```python
from build123d import *

# Parameters (mm, degrees)
SKETCH1_R           = 1.5
SKETCH1_R_2         = 1.7
SKETCH1_R_3         = 2
SKETCH1_W           = 32
SKETCH1_H           = 15
BOSS_EXTRUDE1_DEPTH = 10


with BuildPart() as part:
    # Sketch1 → Boss-Extrude1 (new body)
    with BuildSketch(Plane.XY):
        Polygon((-86.049704166, 116.333921241), (48.950295834, 116.333921241), (48.950295834, 81.333921241), (56.950295834, 81.333921241), (56.950295834, 79.313921241), (130.950295834, 79.313921241), (130.950295834, 81.333921241), (138.950295834, 81.333921241), (138.950295834, 116.333921241), (273.950295834, 116.333921241), (273.950295834, -113.666078759), (138.950295834, -113.666078759), (138.950295834, -78.666078759), (130.950295834, -78.666078759), (130.950295834, -76.646078759), (56.950295834, -76.646078759), (56.950295834, -78.666078759), (48.950295834, -78.666078759), (48.950295834, -113.666078759), (-86.049704166, -113.666078759), (-86.049704166, -78.666078759), (33.950295834, -78.666078759), (33.950295834, 81.333921241), (-86.049704166, 81.333921241), align=None)
        with Locations((63.950295834, 72.313921241)):
            Circle(SKETCH1_R, mode=Mode.SUBTRACT)
        with Locations((63.950295834, 61.313921241)):
            Circle(SKETCH1_R, mode=Mode.SUBTRACT)
        with Locations(Location((123.950295834, 72.313921241, 0), (0, 0, 180))):
            Circle(SKETCH1_R, mode=Mode.SUBTRACT)
        with Locations(Location((123.950295834, 61.313921241, 0), (0, 0, 180))):
            Circle(SKETCH1_R, mode=Mode.SUBTRACT)
        with Locations(Location((63.950295834, -69.646078759, 0), (0, 0, 180))):
            Circle(SKETCH1_R, mode=Mode.SUBTRACT)
        with Locations(Location((63.950295834, -58.646078759, 0), (0, 0, 180))):
            Circle(SKETCH1_R, mode=Mode.SUBTRACT)
        with Locations((123.950295834, -69.646078759)):
            Circle(SKETCH1_R, mode=Mode.SUBTRACT)
        with Locations((123.950295834, -58.646078759)):
            Circle(SKETCH1_R, mode=Mode.SUBTRACT)
        with Locations((-44.099704166, -96.166078759)):
            Circle(SKETCH1_R_2, mode=Mode.SUBTRACT)
        with Locations(Location((-37.999704166, -96.166078759, 0), (0, 0, 180))):
            Circle(SKETCH1_R_2, mode=Mode.SUBTRACT)
        with Locations(Location((-44.099704166, 98.833921241, 0), (0, 0, 180))):
            Circle(SKETCH1_R_2, mode=Mode.SUBTRACT)
        with Locations((-37.999704166, 98.833921241)):
            Circle(SKETCH1_R_2, mode=Mode.SUBTRACT)
        with Locations(Location((232.000295834, -96.166078759, 0), (0, 0, 180))):
            Circle(SKETCH1_R_2, mode=Mode.SUBTRACT)
        with Locations((225.900295834, -96.166078759)):
            Circle(SKETCH1_R_2, mode=Mode.SUBTRACT)
        with Locations(Location((225.900295834, 98.833921241, 0), (0, 0, 180))):
            Circle(SKETCH1_R_2, mode=Mode.SUBTRACT)
        with Locations((232.000295834, 98.833921241)):
            Circle(SKETCH1_R_2, mode=Mode.SUBTRACT)
        with Locations((82.718725704, 1.333921241)):
            Circle(SKETCH1_R_3, mode=Mode.SUBTRACT)
        with Locations((207.29497673, 1.333921241)):
            Circle(SKETCH1_R_3, mode=Mode.SUBTRACT)
        with Locations((263.950295834, 1.333921241)):
            Circle(SKETCH1_R_3, mode=Mode.SUBTRACT)
        with Locations((238.950295834, 1.333921241)):
            Rectangle(SKETCH1_W, SKETCH1_H, mode=Mode.SUBTRACT)
    extrude(amount=BOSS_EXTRUDE1_DEPTH)


solid = part.part
```
Here's how the part is built. I have some questions about the finished solid (model axes, mm). A direction names the side the tool comes from. Coordinates: 2 decimals unless noted, no trailing zeros. Order: outer loops, then holes, each group sorted by start corner. A loop starts at its lowest first (then second) coordinate and runs counter-clockwise, first axis right, second up. Notation, with made-up numbers: (17.5, -13.75) -> (52.5, -13.75) arc R21 cw to (52.5, 3.25) -> close; hole circle Ø2 at (13, 26.25). An arc over 180 degrees is marked (long way). Return JSON: item names as keys, results as strings.
1) On a 3-axis mill with a long thin cutter (end or side, diameter ignored), from which of +Z, -Z, +X, -X, +Y, -Y can I reach the whole of each face in a straight line? I mean faces 1 (the flat face through (138.95, 99, 5)), 2 (the flat face through (-25, 81.334, 5)), 3 (the flat face through (94, -76.646, 5)). Say none if no direction works.
Conclusion:
{"face 1": "+Z, -Z, +Y", "face 2": "+Z, -Z, -X", "face 3": "+Z, -Z, -Y"}
2) If I drill on probe 1 along X at (y, z) = (95, 5); probe 2 along X at (y, z) = (6.5, 4.5); probe 3 along Y at (x, z) = (-56, 2.5), over which ranges is the centre line in solid material (lowest first)?
Conclusion:
{"probe 1": "x = -86.05 to 48.95, 138.95 to 273.95", "probe 2": "x = 33.95 to 222.95, 254.95 to 273.95", "probe 3": "y = -113.67 to -78.67, 81.33 to 116.33"}
3) If we section it at D-D on z = 8.5: State how many separate pieces and enclosed holes the cut face has, plus the area to 3 significant figures.
Conclusion:
{"separate pieces": "1", "enclosed holes": "20", "area": "56,400 mm²"}
4) If we section it at A-A on x = 9: List the corners of the cut face in (y, z) for me, plus the area to 3 significant figures.
Conclusion:
{"outline": "(-113.67, 0) -> (-78.67, 0) -> (-78.67, 10) -> (-113.67, 10) -> close; (81.33, 0) -> (116.33, 0) -> (116.33, 10) -> (81.33, 10) -> close", "area": "700 mm²"}
5) If we section it at B-B on y = 90.5: List the corners of the cut face in (x, z) for me, plus the area to 3 significant figures.
Conclusion:
{"outline": "(-86.05, 0) -> (48.95, 0) -> (48.95, 10) -> (-86.05, 10) -> close; (138.95, 0) -> (273.95, 0) -> (273.95, 10) -> (138.95, 10) -> close", "area": "2,700 mm²"}
6) If we section it at C-C on y = -24.5: List the corners of the cut face in (x, z) for me.
Conclusion:
{"outline": "(33.95, 0) -> (273.95, 0) -> (273.95, 10) -> (33.95, 10) -> close"}
7) I'm going to push flat-ended pins straight in: P1, Ø1.5, axis at x = 67.5, z = 2.5, coming from the +Y side; P2, Ø5, axis at y = -36.5, z = 6.5, coming from the -X side; P3, Ø2.5, axis at x = 123.95, y = -58.65, coming from the +Z side; P4, Ø4, axis at x = 53, z = 7.5, coming from the +Y side. Where does each tip first touch, or does it pass through?
Conclusion:
{"P1": "stops at y = 79.31", "P2": "stops at x = 33.95", "P3": "passes through", "P4": "stops at y = 81.33"}
